Could you check a few things on this model? Use its own coordinates, in mm. A direction names the side the tool comes from. Round coordinates to 2 decimals unless told otherwise and drop trailing zeros. Write each loop counter-clockwise with the first axis right and the second up, starting at its lowest first coordinate (ties: lowest second). Pieces come first, ordered by that corner, then holes. Notation, with made-up numbers: (25, 80) -> (30, 80) arc R18 ccw to (30, 106) -> close; hole circle Ø2 at (-28, 12.25). An arc over 180 degrees is marked (long way). Answer in a Markdown table with one row per item. Add a question column.
```python
from build123d import *

# Parameters (mm, degrees)
F2_R   = 26.9875
F2_R_2 = 18.8595


with BuildPart() as f3:
    # F3: sweep along a path in F0
    with BuildLine(Plane.YZ) as f3_path:
        Line((2438.4, 0), (125.4125, 0))
        ThreePointArc((125.4125, 0), (36.732471, 36.732471), (0, 125.4125))
        Line((0, 125.4125), (0, 609.6))
    # F2 (on plane+point) → F3 (sweep)
    with BuildSketch(Plane.XZ.offset(-2438.4)):
        Circle(F2_R)
        Circle(F2_R_2, mode=Mode.SUBTRACT)
    sweep(path=f3_path.line)


solid = f3.part
```
(1) On a 3-axis mill with a long thin cutter (end or side, diameter ignored), from which of +Z, -Z, +X, -X, +Y, -Y can I reach the whole of each face in a straight line? I mean faces 1 (the face through (-19.89, 1265.72, 18.24)), 2 (the face through (18.4, 2438.4, -5.6)). Say none if no direction works.
(2) Suppose I cut it at A-A, the plane y = 2164.5. Please give me the cut outline in (x, z) (1 decimal).
(3) For P1, Ø1, axis at x = -15, z = 125, coming from the +Y side; P2, Ø12, axis at x = 0, y = 1574, coming from the +Z side; P3, Ø10, axis at x = 12, y = 1064, coming from the -Z side, each with a flat end and sliding along its axis, tell me the tip position at first contact or that it passes through.
(4) I need wall thicknesses on L1, parallel to Y at x = -2, z = 542; L2, parallel to Y at x = -4, z = 351; L3, parallel to Z at x = 0, y = 1648. Which ranges of each line are inside material? Lowest first, please.
Response:
| question | item | result |
|---|---|---|
| 1 | face 1 | +Y |
| 1 | face 2 | +Z, -Z, +X, -X, +Y |
| 2 | outline | circle Ø54 at (0, 0); hole circle Ø37.7 at (0, 0) |
| 3 | P1 | y = 22.76 |
| 3 | P2 | z = 26.99 |
| 3 | P3 | z = -26.06 |
| 4 | L1 | -26.91 to -18.75, 18.75 to 26.91 |
| 4 | L2 | -26.69 to -18.43, 18.43 to 26.69 |
| 4 | L3 | -26.99 to -18.86, 18.86 to 26.99 |
